Autodesk Inventor part; units mm, degrees
ref_plane "YZ Plane" through (0, 0, 0) normal (1, 0, 0) x (0, 1, 0)
ref_plane "XZ Plane" through (0, 0, 0) normal (0, 1, 0) x (-1, 0, 0)
ref_plane "XY Plane" through (0, 0, 0) normal (0, 0, 1) x (1, 0, 0)
sketch "Sketch3" plane through (0, 0, 0) normal (0, 1, 0) x (-1, 0, 0)
  line L0 (2.5, 12) -> (-2.5, 12)
  line L1 (-2.5, 12) -> (-2.5, -12)
  line L2 (-2.5, -12) -> (2.5, -12)
  line L3 (2.5, -12) -> (2.5, 12)
  point P0 (0, 0)
  point P1 (0, 12)
  point P2 (2.5, 0)
  dimension "d6" = 5
  dimension "d7" = 24
extrude "Extrusion3" add sketch "Sketch3" along normal blind 62
sketch "Sketch4" plane through (2.5, 0, 12) normal (1, 0, 0) x (0, 0, -1)
  line L0 (0, 62) -> (24, 62)
  line L1 (24, 62) -> (24, 57)
  line L2 (24, 57) -> (0, 57)
  line L3 (0, 57) -> (0, 62)
  line L4 (0, 5) -> (24, 5)
  line L5 (24, 5) -> (24, 0)
  line L6 (24, 0) -> (0, 0)
  line L7 (0, 0) -> (0, 5)
  line L8 (0, 62) -> (24, 62)
  line L9 (0, 0) -> (24, 0)
  line L10 (0, 0) -> (0, 62)
  point P0 (12, 0)
  point P1 (12, 62)
  point P2 (12, 0)
  point P3 (12, 57)
  point P4 (12, 62)
  point P5 (12, 5)
  point P6 (12, 0)
  point P7 (0, 59.5)
  dimension "d10" = 5
extrude "Extrusion4" add sketch "Sketch4" along normal blind 40 and the other way blind 45
fillet "Fillet4" radius 12 8 edges at (42.5, 2.5, -12) (42.5, 2.5, 12) (42.5, 59.5, 12) (42.5, 59.5, -12) (-42.5, 59.5, 12) (-42.5, 2.5, 12) (-42.5, 59.5, -12) (-42.5, 2.5, -12)
sketch "Sketch8" plane through (0, 62, 0) normal (0, 1, 0) x (1, 0, 0)
  circle A0 centre (-30.5, 0) radius 3.75
  circle A1 centre (30.5, 0) radius 3.75
  arc A2 (-30.5, 12) -> (-30.5, -12) centre (-30.5, 0) ccw
  arc A3 (30.5, -12) -> (30.5, 12) centre (30.5, 0) ccw
  point P0 (0, 0)
  dimension "d27" = 7.5
extrude "Extrusion7" cut sketch "Sketch8" against normal up to surface (5 mm away)
sketch "Sketch9" plane through (0, 0, 0) normal (0, -1, 0) x (1, 0, 0)
  circle A0 centre (-30.5, 0) radius 6.5
  circle A1 centre (30.5, 0) radius 6.5
  arc A2 (-30.5, 12) -> (-30.5, -12) centre (-30.5, 0) ccw
  arc A3 (30.5, -12) -> (30.5, 12) centre (30.5, 0) ccw
  point P0 (0, 0)
  dimension "d30" = 13
extrude "Extrusion8" cut sketch "Sketch9" against normal up to next
equation "\"d6\" = b_mat_thickness"
equation "\"d7\" = sa_diameter"
equation "\"d10\" = b_mat_thickness"
equation "\"d24\" = d11 + b_mat_thickness"
equation "\"d26\" = 0.5 * sa_diameter"
equation "\"d30\" = bb_outer_diameter"
properties part number "Middle_leg"
The listing builds one solid part. Answer for the finished solid, in the listing's coordinates (mm). A direction names the side the tool comes from. Round coordinates to 2 decimals unless told otherwise and drop trailing zeros. Write each loop counter-clockwise with the first axis right and the second up, starting at its lowest first coordinate (ties: lowest second). Pieces come first, ordered by that corner, then holes. Notation, with made-up numbers: (76, -26.5) -> (126, -26.5) arc R20 cw to (126, -3.5) -> close; hole circle Ø6 at (-31.5, 35.25). An arc over 180 degrees is marked (long way). Use CSV: the item, a comma, the result in double quotes. Start each with the question number.
(1) Which of the six approach directions +Z, -Z, +X, -X, +Y, -Y give full straight-line access (tool end or side, diameter ignored) to faces 1 (the face through (-23, 57, 0)), 2 (the face through (-37, 2, 0)), 3 (the face through (2.5, 31, 0))?
(2) Consider L1, parallel to X at y = 58.2, z = 0; L2, parallel to Z at x = 30.5, y = 58.75; L3, parallel to Y at x = 7, z = -2. Determine where each line is inside the solid, lowest interval first. Write a range as from..to.
(3) Section D-D on y = 32 is taken. Give the vertices of the cut face in (x, z), then the cut area to 3 significant figures.
(4) Section A-A on x = 19.5 is taken. Give the vertices of the cut face in (y, z), then the cut area to 3 significant figures.
(5) Section B-B on z = 1.75 is taken. Give the vertices of the cut face in (x, y).
(6) The mould has two halves that part along X. Classify faces 4 (the face through (24, 2, 0)), 5 (the face through (38.89, 59.54, 8.58)), 6 (the face through (22, 57, 0)): released by +X, released by -X, zero draft, split by the parting line, or undercut.
(7) Section C-C on x = 28 is taken. Give the vertices of the cut face in (y, z).
(8) Each of these flat-tipped pins is pushed along its axis until it touches: pin 1 (10 mm diameter, centred on x = -30.5, z = 0, fed in from -Y); pin 2 (2 mm diameter, centred on y = 30, z = -9, fed in from +X); pin 3 (3 mm diameter, centred on y = 9.5, z = 1.5, fed in from -X). Where does it stop, or does it pass through?
A:
1,face 1,"+Z, -Z, -X"
1,face 2,"-Y"
1,face 3,"+Z, -Z, +X"
2,L1,"x = -42.5..-34.25, -26.75..26.75, 34.25..42.5"
2,L2,"z = -12..-3.75, 3.75..12"
2,L3,"y = 0..5, 57..62"
3,outline,"(-2.5, -12) -> (2.5, -12) -> (2.5, 12) -> (-2.5, 12) -> close"
3,area,"120 mm²"
4,outline,"(0, -12) -> (5, -12) -> (5, 12) -> (0, 12) -> close; (57, -12) -> (62, -12) -> (62, 12) -> (57, 12) -> close"
4,area,"240 mm²"
5,outline,"(-42.37, 0) -> (-36.76, 0) -> (-36.76, 5) -> (-42.37, 5) -> close; (-42.37, 57) -> (-33.82, 57) -> (-33.82, 62) -> (-42.37, 62) -> close; (-27.18, 57) -> (-2.5, 57) -> (-2.5, 5) -> (-24.24, 5) -> (-24.24, 0) -> (24.24, 0) -> (24.24, 5) -> (2.5, 5) -> (2.5, 57) -> (27.18, 57) -> (27.18, 62) -> (-27.18, 62) -> close; (33.82, 57) -> (42.37, 57) -> (42.37, 62) -> (33.82, 62) -> close; (36.76, 0) -> (42.37, 0) -> (42.37, 5) -> (36.76, 5) -> close"
6,face 4,"undercut"
6,face 5,"released by +X"
6,face 6,"zero draft"
7,outline,"(0, -12) -> (5, -12) -> (5, -6) -> (0, -6) -> close; (0, 6) -> (5, 6) -> (5, 12) -> (0, 12) -> close; (57, -12) -> (62, -12) -> (62, -2.8) -> (57, -2.8) -> close; (57, 2.8) -> (62, 2.8) -> (62, 12) -> (57, 12) -> close"
8,pin 1,"stops at y = 57"
8,pin 2,"stops at x = 2.5"
8,pin 3,"stops at x = -2.5"
